Could you check a few things on this model? Use its own coordinates, in mm. Coordinates: 2 decimals unless noted, no trailing zeros. Write each loop counter-clockwise with the first axis right and the second up, starting at its lowest first coordinate (ties: lowest second). Pieces come first, ordered by that corner, then holes.
```python
from build123d import *

# Parameters (mm, degrees)
SKETCH_1_R          = 2.1
EXTRUDE_1_DEPTH     = 4
CUT_EXTRUDE_2_DEPTH = 13
SKETCH_8_R          = 2.1
CUT_EXTRUDE_3_DEPTH = 4
SKETCH_9_W          = 4
SKETCH_9_H          = 200
EXTRUDE_4_DEPTH     = 4
FILLET_2_R          = 10
SKETCH_10_W         = 25
SKETCH_10_H         = 40
SKETCH_10_W_2       = 21
SKETCH_10_H_2       = 21
CUT_EXTRUDE_5_DEPTH = 13
FILLET_3_R          = 2
FILLET_4_R          = 3


with BuildPart() as part:
    # 草图1 → 凸台-拉伸1 (new body)
    with BuildSketch(Plane.XY):
        Polygon((-20, 100), (-77, 55), (-77, -55), (-20, -100), (20, -100), (20, 100), align=None)
        with Locations((-72, 47.5)):
            Circle(SKETCH_1_R, mode=Mode.SUBTRACT)
        with Locations((-47, 47.5)):
            Circle(SKETCH_1_R, mode=Mode.SUBTRACT)
        with Locations((-72, -47.5)):
            Circle(SKETCH_1_R, mode=Mode.SUBTRACT)
        with Locations((-47, -47.5)):
            Circle(SKETCH_1_R, mode=Mode.SUBTRACT)
        with Locations((-16, -66)):
            Circle(SKETCH_1_R, mode=Mode.SUBTRACT)
        with Locations((-16, -94)):
            Circle(SKETCH_1_R, mode=Mode.SUBTRACT)
        with Locations((-16, 94)):
            Circle(SKETCH_1_R, mode=Mode.SUBTRACT)
        with Locations((-16, 66)):
            Circle(SKETCH_1_R, mode=Mode.SUBTRACT)
    extrude(amount=EXTRUDE_1_DEPTH)

    # 草图6 → 切除-拉伸2 (cut)
    with BuildSketch(Plane(origin=(0, 0, 0), x_dir=(-1, 0, 0), z_dir=(0, 0, -1))):
        with BuildLine():
            Line((20, 100), (75.306183573, 51.250886586))
            ThreePointArc((75.306183573, 51.250886586), (76.556913312, 49.557800055), (77, 47.5))
            Line((77, 47.5), (77, 55))
            Line((77, 55), (20, 100))
        make_face()
        with BuildLine():
            Line((77, -55), (77, -47.5))
            ThreePointArc((77, -47.5), (76.556913312, -49.557800055), (75.306183573, -51.250886586))
            Line((75.306183573, -51.250886586), (20, -100))
            Line((20, -100), (77, -55))
        make_face()
    extrude(amount=-CUT_EXTRUDE_2_DEPTH, mode=Mode.SUBTRACT)

    # 草图8 → 切除-拉伸3 (cut)
    with BuildSketch(Plane.XY.offset(4)):
        with Locations((12, 94)):
            Circle(SKETCH_8_R)
        with Locations((12, 66)):
            Circle(SKETCH_8_R)
        with Locations((12, -66)):
            Circle(SKETCH_8_R)
        with Locations((12, -94)):
            Circle(SKETCH_8_R)
    extrude(amount=-CUT_EXTRUDE_3_DEPTH, mode=Mode.SUBTRACT)

    # 草图9 → 凸台-拉伸4 (add)
    with BuildSketch(Plane.XY.offset(4)):
        with Locations((18, 0)):
            Rectangle(SKETCH_9_W, SKETCH_9_H)
    extrude(amount=-EXTRUDE_4_DEPTH)

    # 圆角2
    fillet_2_edges = [part.edges().sort_by_distance(p)[0] for p in [
        (-20, 100, 2),
        (-20, -100, 2),
    ]]
    fillet(fillet_2_edges, radius=FILLET_2_R)

    # 草图10 → 切除-拉伸5 (cut)
    with BuildSketch(Plane.XY.offset(4)):
        Polygon((8.756169307, 62), (-17.741713503, 62), (-30.169479576, 51.045662914), (-12.959361551, 9.201454384), align=None)
        Polygon((-17.284469142, -1.314493483), (-36.518131022, 45.449704029), (-39, 43.262084048), (-39, -43.262084048), (-35.724549591, -46.14919889), align=None)
        Polygon((12, 54.113039099), (-9.715530858, 1.314493483), (12, -51.484052132), align=None)
        Polygon((7.674892409, -62), (-14.040638449, -9.201454384), (-30.963061007, -50.346168054), (-17.741713503, -62), align=None)
        with Locations((-59.5, -22.5)):
            Rectangle(SKETCH_10_W, SKETCH_10_H)
        with Locations((-59.5, 22.5)):
            Rectangle(SKETCH_10_W, SKETCH_10_H)
        Polygon((-43.642701965, 52.5), (-21, 72.458195897), (-21, 92.453468554), (-66.327467753, 52.5), align=None)
        with Locations((-2, 80)):
            Rectangle(SKETCH_10_W_2, SKETCH_10_H_2)
        Polygon((-21, -72.458195897), (-21, -92.453468554), (-66.327467753, -52.5), (-43.642701965, -52.5), align=None)
        with Locations((-2, -80)):
            Rectangle(SKETCH_10_W_2, SKETCH_10_H_2)
    extrude(amount=-CUT_EXTRUDE_5_DEPTH, mode=Mode.SUBTRACT)

    # 圆角3
    # the kernel refuses this fillet: 2 mm, written as the material it adds along each edge
    with BuildSketch(Plane(origin=(-35.724549591, -46.14919889, 4), x_dir=(0.3803746509932158, 0.9248324847678034, 0), z_dir=(0, 0, -1))) as fillet_3_piece_1:
        with BuildLine():
            CenterArc((FILLET_3_R * 1.4029157826, -FILLET_3_R), FILLET_3_R, 90, 109.037368678)
            Line((FILLET_3_R * 0.457609745735, -FILLET_3_R * 1.3261847585), (0, 0))
            Line((0, 0), (FILLET_3_R * 1.4029157826, 0))
        make_face()
    extrude(amount=4)
    with BuildSketch(Plane(origin=(-39, -43.262084048, 4), x_dir=(0, 1, 0), z_dir=(0, 0, -1)), Plane(origin=(-39, 43.262084048, 4), x_dir=(0.7501773172639279, 0.6612367145453253, 0), z_dir=(0, 0, -1))) as fillet_3_piece_2:
        with BuildLine():
            CenterArc((FILLET_3_R * 0.451577617263, FILLET_3_R), FILLET_3_R, 221.394260007, 48.605739993)
            Line((-FILLET_3_R * 0.298599700001, FILLET_3_R * 0.338763285455), (0, 0))
            Line((0, 0), (FILLET_3_R * 0.451577617263, 0))
        make_face()
    extrude(amount=4)
    with BuildSketch(Plane(origin=(-36.518131022, 45.449704029, 4), x_dir=(0.3803746509932163, -0.9248324847678032, 0), z_dir=(0, 0, -1))) as fillet_3_piece_3:
        with BuildLine():
            CenterArc((FILLET_3_R * 1.4029157826, FILLET_3_R), FILLET_3_R, 160.962631322, 109.037368678)
            Line((FILLET_3_R * 0.457609745735, FILLET_3_R * 1.3261847585), (0, 0))
            Line((0, 0), (FILLET_3_R * 1.4029157826, 0))
        make_face()
    extrude(amount=4)

    # 圆角4
    fillet_4_edges = [part.edges().sort_by_distance(p)[0] for p in [
        (-47, 2.5, 2),
        (-72, 2.5, 2),
        (-72, 42.5, 2),
        (-47, 42.5, 2),
        (-21, 72.458195897, 2),
        (-43.642701965, 52.5, 2),
        (-66.327467753, 52.5, 2),
        (-21, 92.453468554, 2),
        (8.5, 69.5, 2),
        (-12.5, 69.5, 2),
        (-12.5, 90.5, 2),
        (8.5, 90.5, 2),
        (-21, -72.458195897, 2),
        (-21, -92.453468554, 2),
        (-66.327467753, -52.5, 2),
        (-43.642701965, -52.5, 2),
        (-17.284469142, -1.314493483, 2),
        (-9.715530858, 1.314493483, 2),
        (-14.040638449, -9.201454384, 2),
        (7.674892409, -62, 2),
        (-17.741713503, -62, 2),
        (-30.963061007, -50.346168054, 2),
        (-47, -42.5, 2),
        (-72, -42.5, 2),
        (-72, -2.5, 2),
        (-47, -2.5, 2),
        (-12.5, -69.5, 2),
        (8.5, -69.5, 2),
        (8.5, -90.5, 2),
        (-12.5, -90.5, 2),
        (8.756169307, 62, 2),
        (-12.959361551, 9.201454384, 2),
        (-30.169479576, 51.045662914, 2),
        (-17.741713503, 62, 2),
    ]]
    fillet(fillet_4_edges, radius=FILLET_4_R)


solid = part.part
```
1. I want a section at B-B on y = -76. Please give me the cut outline in (x, z), plus the area to 3 significant figures.
Verdict:
outline: (-47.23, 0) - (-39.67, 0) - (-39.67, 4) - (-47.23, 4) - close; (-21, 0) - (-12.5, 0) - (-12.5, 4) - (-21, 4) - close; (8.5, 0) - (20, 0) - (20, 4) - (8.5, 4) - close
area: 110 mm2
2. For pin 1 (10 mm diameter, centred on x = -66.5, y = -42, fed in from -Z); pin 2 (2 mm diameter, centred on x = -55, z = 1.5, fed in from +Y); pin 3 (4 mm diameter, centred on x = -16, y = 94, fed in from +Z); pin 4 (2 mm diameter, centred on y = 75.5, z = 1.5, fed in from -X), each with a flat end and sliding along its axis, tell me the tip position at first contact or that it passes through.
Verdict:
pin 1: stops at z = 0
pin 2: stops at y = 70.03
pin 3: passes through
pin 4: stops at x = -48.93
3. I want a section at C-C on z = 0.8. Give the number of separate pieces and of enclosed holes in the cut face, plus the area to 3 significant figures.
Verdict:
separate pieces: 1
enclosed holes: 22
area: 7,880 mm2
4. Please list where these lines run through material, in increasing order: line 1 along X through (y, z) = (-31, 0.45); line 2 along X through (y, z) = (-18, 0.9); line 3 along X through (y, z) = (-10, 3.1).
Verdict:
line 1: x = -77 to -72, -47 to -39, -29.49 to -23.01, -5.08 to 3.58, 12 to 20
line 2: x = -77 to -72, -47 to -39, -24.15 to -17.66, -10.42 to -1.77, 12 to 20
line 3: x = -77 to -72, -47 to -39, -20.86 to -5.06, 12 to 20
5. I want a section at A-A on y = 10. Please give me the cut outline in (x, z), plus the area to 3 significant figures.
Verdict:
outline: (-77, 0) - (-72, 0) - (-72, 4) - (-77, 4) - close; (-47, 0) - (-39, 0) - (-39, 4) - (-47, 4) - close; (-21.94, 0) - (-6.14, 0) - (-6.14, 4) - (-21.94, 4) - close; (12, 0) - (20, 0) - (20, 4) - (12, 4) - close
area: 147 mm2
6. If we mould it in two halves opening along X, with no side actions, what happens to faces 1 (the face through (-73.666, 46.222, 1.972)), 2 (the face through (-76.545, 49.585, 1.972)), 3 (the face through (-60, -42.5, 2))? For each: pulls with the +X half, pulls with the -X half, needs draft (parallel to the pull), parting line crosses it, or undercut.
Verdict:
face 1: undercut
face 2: pulls with the -X half
face 3: undercut
